from build123d import *

# Parameters (mm, degrees)
SKETCH1_R           = 6
SKETCH1_R_2         = 2
BOSS_EXTRUDE1_DEPTH = 2
FILLET1_R           = 1.5


with BuildPart() as part:
    # Sketch1 → Boss-Extrude1 (new body)
    with BuildSketch(Plane.XY):
        with Locations((-174.416251328, -25.172160385)):
            Circle(SKETCH1_R)
        with Locations((-174.416251328, -25.172160385)):
            Circle(SKETCH1_R_2, mode=Mode.SUBTRACT)
        with BuildLine():
            ThreePointArc((-170.173610641, -29.414801072), (-173.850108495, -31.145390859), (-177.78627055, -30.13632904))
            Line((-177.78627055, -30.13632904), (-179.432101814, -36.199979912))
            ThreePointArc((-179.432101814, -36.199979912), (-174.407079396, -33.853814689), (-168.876035514, -34.257417374))
            Line((-168.876035514, -34.257417374), (-170.173610641, -29.414801072))
        make_face()
    extrude(amount=BOSS_EXTRUDE1_DEPTH)

    # Fillet1
    fillet1_edges = [part.edges().sort_by_distance(p)[0] for p in [
        (-168.876035514, -34.257417374, 1),
        (-179.432101814, -36.199979912, 1),
    ]]
    fillet(fillet1_edges, radius=FILLET1_R)


solid = part.part
The model under review builds one solid part; all positions refer to its coordinate system, in mm. A direction names the side the tool comes from. Round coordinates to 2 decimals unless told otherwise and drop trailing zeros. Loops run counter-clockwise (first coordinate to the right, second up) from the corner with the lowest first, then second, coordinate; pieces in that order, holes last. Notation, with made-up numbers: M 67.25,23 L 88.25,23 A29 cw 88.25,60 Z; hole C 86.25,16.25 d9. An arc over 180 degrees is marked long. Answer as a JSON object with one key per item and string values.
Item 1: We need section B-B, the plane y = -24.5. State the section outline as (x, z) points.
Check sheet entries:
{"outline": "M -180.38,0 L -176.3,0 L -176.3,2 L -180.38,2 Z; M -172.53,0 L -168.45,0 L -168.45,2 L -172.53,2 Z"}
Item 2: Tool access review of faces 4 (the face through (-173.89, -33.77, 0.99)), 5 (the face through (-169.84, -30.66, 0.99)): name each direction out of +Z, -Z, +X, -X, +Y, -Y from which nothing blocks a thin tool from reaching the whole face with its end or side.
Check sheet entries:
{"face 4": "+Z, -Z, -Y", "face 5": "+Z, -Z, +X"}
Item 3: We need section C-C, the plane z = 1.6. State the section outline as (x, y) points, and give its area (3 significant figures).
Check sheet entries:
{"outline": "M -178.47,-32.66 A1.5 ccw -176.47,-34.45 A11 cw -171.14,-33.75 A1.5 ccw -169.52,-31.87 L -170.17,-29.41 A6 ccw long -177.79,-30.14 Z; hole C -174.42,-25.17 d4", "area": "129 mm2"}
Item 4: The part is to be moulded in two halves that separate along X. For faces 1 (the face through (-174.85, -27.125, 0.986)), 2 (the face through (-173, -27, 2)), 3 (the face through (-178.124, -31.38, 0.986)), say which applies: +X half, -X half, draft (parallel to the pull), parting line (faces both ways), or undercut.
Check sheet entries:
{"face 1": "undercut", "face 2": "draft", "face 3": "-X half"}
Item 5: Clearance check with a flat-ended pin moving along its axis: P1, Ø2.5, axis at x = -174.42, y = -25.17, coming from the -Z side. State where the tip first meets the part, or that it passes through.
Check sheet entries:
{"P1": "through"}
Item 6: We need section A-A, the plane x = -175.5. State the section outline as (y, z) points, and give its area (3 significant figures).
Check sheet entries:
{"outline": "M -34.11,0 L -26.85,0 L -26.85,2 L -34.11,2 Z; M -23.49,0 L -19.27,0 L -19.27,2 L -23.49,2 Z", "area": "23.0 mm2"}
Item 7: For line 1 along X through (y, z) = (-25.25, 0.7); line 2 along Y through (x, z) = (-175, 0.35); line 3 along Y through (x, z) = (-175.25, 0.2), list the stretches that pass through material, from the lowest coordinate up.
Check sheet entries:
{"line 1": "-180.42 to -176.41, -172.42 to -168.42", "line 2": "-33.98 to -27.09, -23.26 to -19.2", "line 3": "-34.04 to -26.99, -23.35 to -19.23"}
Item 8: We need section D-D, the plane y = -32.5. State the section outline as (x, z) points.
Check sheet entries:
{"outline": "M -178.43,0 L -169.48,0 L -169.48,2 L -178.43,2 Z"}
